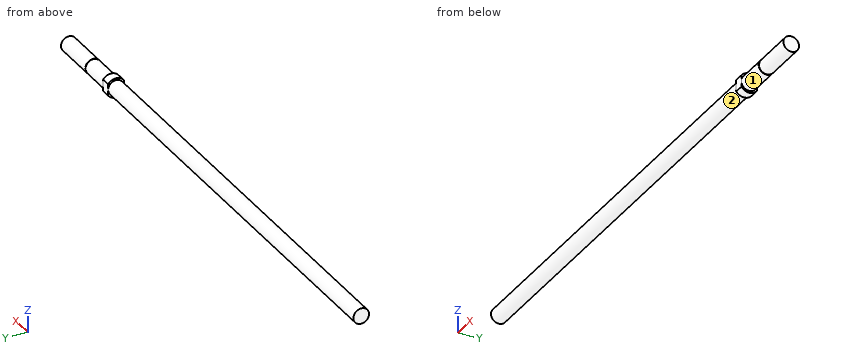
from build123d import *

# Parameters (mm, degrees)
SKETCH2_OUTSIDE_W   = 54.09
SKETCH2_OUTSIDE_H   = 54.09
SKETCH2_OUTSIDE_W_2 = 7.9375
SKETCH2_OUTSIDE_H_2 = 6.35
CUT_EXTRUDE1_DEPTH  = 221.472


with BuildPart() as part:
    # Sketch1 → Revolve1 (revolve)
    with BuildSketch(Plane.XY):
        Polygon((0, 0), (-220.472, 0), (-220.472, 3.175), (-35.56, 3.175), (-35.56, 3.96875), (-31.75, 3.96875), (-31.75, 3.175), (-18.669, 3.175), (-18.669, 3.0226), (-18.288, 3.0226), (-18.288, 3.175), (0, 3.175), align=None)
    revolve(axis=Axis((0, 0, 0), (-1, 0, 0)))

    # Sketch2 outside → Cut-Extrude1 (cut, through all)
    with BuildSketch(Plane(origin=(0, 0, 0), x_dir=(0, 0, -1), z_dir=(1, 0, 0))):
        Rectangle(SKETCH2_OUTSIDE_W, SKETCH2_OUTSIDE_H)
        Rectangle(SKETCH2_OUTSIDE_W_2, SKETCH2_OUTSIDE_H_2, mode=Mode.SUBTRACT)
    extrude(amount=-CUT_EXTRUDE1_DEPTH, mode=Mode.SUBTRACT)


solid = part.part
Could you check a few things on this model? Use its own coordinates, in mm. Face numbers are marked on the shaded views. A direction names the side the tool comes from. Give positions to 0.01 mm unless a question says otherwise; leave off trailing zeros. Write each loop counter-clockwise with the first axis right and the second up, starting at its lowest first coordinate (ties: lowest second). Pieces come first, ordered by that corner, then holes. Notation, with made-up numbers: (-13, 42) -> (-4, 42) arc R14 cw to (-4, 46) -> close; hole circle Ø9 at (15, 42). An arc over 180 degrees is marked (long way). Write each question's results on one line, items separated by ' | '. Start each with the question number.
Q1. Which directions (+Z, -Z, +X, -X, +Y, -Y) give clear straight access to the entire face, cutting with the end or side of a thin tool? Please do the marked faces 1 and 2.
Q2. Suppose I cut it at A-A, the plane y = 0. List the corners of the cut face in (x, z) for me (3 decimals).
Q3. I'm going to push flat-ended pins straight in: pin 1 Ø1 at (x, z) = (-47, -1) entering from -Y; pin 2 Ø3 at (x, y) = (-48, -1.5) entering from +Z (3 decimals); pin 3 Ø1 at (x, z) = (-79, -1.5) entering from +Y. Where does each tip first touch, or does it pass through?
Q4. I need wall thicknesses on probe 1 along Z at (x, y) = (-188, 1); probe 2 along Z at (x, y) = (-55, -0.5); probe 3 along X at (y, z) = (0.5, 3.25). Which ranges of each line are inside material? Lowest first, please.
Q5. Suppose I cut it at B-B, the plane x = -184.5. List the corners of the cut face in (y, z) for me (3 decimals), and give its area (3 significant figures).
Outcome:
1) face 1: +X | face 2: -X
2) outline: (-220.472, -3.175) -> (-35.56, -3.175) -> (-35.56, -3.969) -> (-31.75, -3.969) -> (-31.75, -3.175) -> (-18.669, -3.175) -> (-18.669, -3.023) -> (-18.288, -3.023) -> (-18.288, -3.175) -> (0, -3.175) -> (0, 3.175) -> (-18.288, 3.175) -> (-18.288, 3.023) -> (-18.669, 3.023) -> (-18.669, 3.175) -> (-31.75, 3.175) -> (-31.75, 3.969) -> (-35.56, 3.969) -> (-35.56, 3.175) -> (-220.472, 3.175) -> close
3) pin 1: y = -3.14 | pin 2: z = 3.175 | pin 3: y = 3.01
4) probe 1: -3.01 to 3.01 | probe 2: -3.14 to 3.14 | probe 3: -35.56 to -31.75
5) outline: circle Ø6.35 at (0, 0) | area: 31.7 mm2
